from build123d import *

# Parameters (mm, degrees)
SKETCH6_R           = 9.525
BOSS_EXTRUDE5_DEPTH = 93.6625
BOSS_EXTRUDE6_DEPTH = 6.35
BOSS_EXTRUDE7_DEPTH = 11.1125
SKETCH9_R           = 3.175
BOSS_EXTRUDE8_DEPTH = 19.05
SKETCH11_R          = 3.81
BOSS_EXTRUDE9_DEPTH = 12.7
SKETCH12_R          = 6.35
CUT_EXTRUDE2_DEPTH  = 50.8


with BuildPart() as part:
    # Sketch6 → Boss-Extrude5 (new body)
    with BuildSketch(Plane.XY):
        Circle(SKETCH6_R)
    extrude(amount=BOSS_EXTRUDE5_DEPTH)

    # Sketch7 → Boss-Extrude6 (add)
    with BuildSketch(Plane.XY.offset(93.6625)):
        Polygon((0, 10.998522628), (-9.525, 5.499261314), (-9.525, -5.499261314), (0, -10.998522628), (9.525, -5.499261314), (9.525, 5.499261314), align=None)
    extrude(amount=-BOSS_EXTRUDE6_DEPTH)

    # Sketch8 → Boss-Extrude7 (add)
    with BuildSketch(Plane(origin=(0, 0, 0), x_dir=(-1, 0, 0), z_dir=(0, 0, -1))):
        Polygon((0, 10.998522628), (-9.525, 5.499261314), (-9.525, -5.499261314), (0, -10.998522628), (9.525, -5.499261314), (9.525, 5.499261314), align=None)
    extrude(amount=-BOSS_EXTRUDE7_DEPTH)

    # Sketch9 → Boss-Extrude8 (add, symmetric)
    with BuildSketch(Plane(origin=(0, 0, 0), x_dir=(1, 0, 0), z_dir=(0, 1, 0))):
        with Locations((0, -5.55625)):
            Circle(SKETCH9_R)
    extrude(amount=BOSS_EXTRUDE8_DEPTH, both=True)

    # Sketch11 → Boss-Extrude9 (add, symmetric)
    with BuildSketch(Plane(origin=(0, 0, 0), x_dir=(1, 0, 0), z_dir=(0, 1, 0))):
        with Locations((0, -5.55625)):
            Circle(SKETCH11_R)
    extrude(amount=BOSS_EXTRUDE9_DEPTH, both=True)

    # Sketch12 → Cut-Extrude2 (cut)
    with BuildSketch(Plane(origin=(0, 0, 0), x_dir=(-1, 0, 0), z_dir=(0, 0, -1))):
        Circle(SKETCH12_R)
    extrude(amount=-CUT_EXTRUDE2_DEPTH, mode=Mode.SUBTRACT)


solid = part.part
Input: part model. Units: mm. Frame: model coordinates. A direction names the side the tool comes from. Coordinates: 2 decimals unless noted, no trailing zeros. Order: outer loops, then holes, each group sorted by start corner. A loop starts at its lowest first (then second) coordinate and runs counter-clockwise, first axis right, second up. Notation, with made-up numbers: M 5,1.5 L 57,1.5 A21 cw 57,19.5 Z; hole C -17,55 d9. An arc over 180 degrees is marked long. Answer in a Markdown table with one row per item.
(1) Access query for faces 1 (the flat face through (-4.696, 8.287, 90.532)), 2 (the flat face through (9, 5, 87.312)), 3 (the cylindrical face through (-0.413, -15.831, 2.408)). Directions: +Z, -Z, +X, -X, +Y, -Y. A direction counts if a zero-diameter tool reaches every point of the face in a straight line with its end or side. Return the directions, or none.
Numbers:
| item | result |
|---|---|
| face 1 | +Z, -X, +Y |
| face 2 | +X, +Y |
| face 3 | -Y |
(2) Contact query for flat-ended pins moving along their axis: pin 1 Ø10 at (y, z) = (-10, 45) entering from +X; pin 2 Ø6 at (x, z) = (0, 69) entering from +Y (3 decimals); pin 3 Ø4 at (x, z) = (-7, 28) entering from +Y. Output: stop coordinate, or through.
Numbers:
| item | result |
|---|---|
| pin 1 | stops at x = 8.11 |
| pin 2 | stops at y = 9.525 |
| pin 3 | stops at y = 8.11 |
(3) Section query A-A, the plane z = 49. Output: boundary loops of the cut face in (x, y) (3 decimals).
Numbers:
| item | result |
|---|---|
| outline | C 0,0 d19.05; hole C 0,0 d12.7 |
(4) Material intervals for line 1 (Y direction, x = 0, z = 28) (3 decimals); line 2 (Y direction, x = -1.25, z = 19); line 3 (X direction, y = 5.5, z = 19), sorted ascending. Write a range as [from, to].
Numbers:
| item | result |
|---|---|
| line 1 | y = [-9.525, -6.35], [6.35, 9.525] |
| line 2 | y = [-9.44, -6.23], [6.23, 9.44] |
| line 3 | x = [-7.78, -3.17], [3.17, 7.78] |
(5) Draft query along Z for faces 4 (the flat face through (0, 19.05, 6)), 5 (the cylindrical face through (-7.559, -5.796, 48.679)), 6 (the flat face through (0, 0, 93.662)). Return one class per face: pulls with the +Z half, pulls with the -Z half, needs draft (parallel to the pull), parting line crosses it, or undercut.
Numbers:
| item | result |
|---|---|
| face 4 | needs draft |
| face 5 | undercut |
| face 6 | pulls with the +Z half |
(6) Section query B-B, the plane y = 15.5. Output: boundary loops of the cut face in (x, z) (3 decimals).
Numbers:
| item | result |
|---|---|
| outline | C 0,5.556 d6.35 |
